```python
from build123d import *

# Parameters (mm, degrees)
SKETCH1_W                    = 14
SKETCH1_H                    = 8
SKETCH1_R                    = 2.5
BASE_FLANGE1_DEPTH           = 2
EDGE_FLANGE1_STRIP_W         = 9.4732
EDGE_FLANGE1_STRIP_H         = 2
EDGE_FLANGE1_STRIP_CUT_DEPTH = 8
EDGE_FLANGE1_DEPTH           = 8
EDGE_FLANGE1_PROFILE_W       = 8
EDGE_FLANGE1_PROFILE_H       = 11.2634
EDGE_FLANGE1_PROFILE_R       = 2.5
EDGE_FLANGE1_FLAT_DEPTH      = 2


# Sheet-metal steps are written as plain solids
with BuildPart() as part:
    # Sketch1 → Base-Flange1 (new body)
    with BuildSketch(Plane(origin=(0, 0, 0), x_dir=(1, 0, 0), z_dir=(0, 1, 0))):
        Rectangle(SKETCH1_W, SKETCH1_H)
        with Locations(Location((-2.5, 0, 0), (0, 0, 270))):
            Circle(SKETCH1_R, mode=Mode.SUBTRACT)
    extrude(amount=-BASE_FLANGE1_DEPTH)

    # Edge-Flange1 strip (across the edge) → Edge-Flange1 strip cut (cut)
    with BuildSketch(Plane(origin=(7, 0, 4), x_dir=(-1, 0, 0), z_dir=(0, 0, -1))):
        with Locations((-2, -1)):
            Rectangle(EDGE_FLANGE1_STRIP_W, EDGE_FLANGE1_STRIP_H)
    extrude(amount=EDGE_FLANGE1_STRIP_CUT_DEPTH, mode=Mode.SUBTRACT)

    # Edge-Flange1 bend section (across the edge) → Edge-Flange1 (add)
    with BuildSketch(Plane(origin=(7, 0, 4), x_dir=(-1, 0, 0), z_dir=(0, 0, -1))):
        with BuildLine():
            Line((0, 0.7366), (2, 0.7366))
            ThreePointArc((2, 0.7366), (2.215745145, 0.215745145), (2.7366, 0))
            Line((2.7366, 0), (2.7366, -2))
            ThreePointArc((2.7366, -2), (0.801531583, -1.198468417), (0, 0.7366))
        make_face()
    extrude(amount=EDGE_FLANGE1_DEPTH)

    # Edge-Flange1 profile (on flange) → Edge-Flange1 flat (add)
    with BuildSketch(Plane(origin=(7, 0, 0), x_dir=(0, 0, -1), z_dir=(1, 0, 0))):
        with Locations((0, 6.3683)):
            Rectangle(EDGE_FLANGE1_PROFILE_W, EDGE_FLANGE1_PROFILE_H)
        with Locations((0, 7.5)):
            Circle(EDGE_FLANGE1_PROFILE_R, mode=Mode.SUBTRACT)
    extrude(amount=-EDGE_FLANGE1_FLAT_DEPTH)


solid = part.part
```
Check sheet for the modelled part. Datum: model origin and axes. Units: mm. A direction names the side the tool comes from. Coordinates: 2 decimals unless noted, no trailing zeros. Order: outer loops, then holes, each group sorted by start corner. A loop starts at its lowest first (then second) coordinate and runs counter-clockwise, first axis right, second up. Notation, with made-up numbers: M 14.5,84.25 L 31.5,84.25 A3 ccw 31.5,89.25 Z; hole C 37.25,-21.75 d5. An arc over 180 degrees is marked long. Write each question's results on one line, items separated by ' | '. Start each with the question number.
1. Go/stop test with a flat-tipped pin: P1, Ø3, axis at y = 2, z = 1.5, coming from the -X side. Record where the tip stops, or that it passes through.
2. Cross-section at A-A on z = 0. Record the cut outline in (x, y).
3. Cross-section at B-B on y = 7.5. Record the cut outline in (x, z), and give its area (3 significant figures).
4. Mould release check, pull along X, two halves, no side actions. Record for faces 1 (the face through (6.01, 5.06, 0.54)), 2 (the face through (7, 5, 2)), 3 (the face through (-4.72, -0.99, 1.15)), 4 (the face through (-7, -1, 0)): +X half, -X half, draft (parallel to the pull), parting line (faces both ways), or undercut.
5. Cross-section at D-D on z = -2.75. Record the cut outline in (x, y), and give its area (3 significant figures).
6. Material ranges on probe 1 along Y at (x, z) = (2.25, 2.25); probe 2 along X at (y, z) = (4, 0.25); probe 3 along Y at (x, z) = (6, 0), recorded low to high.
7. Cross-section at C-C on x = -2.5. Record the cut outline in (y, z).
8. Access from +Z, -Z, +X, -X, +Y, -Y to the whole of each face (thin tool, end or side, straight path). Record for faces 5 (the face through (0, 0, -2)), 6 (the face through (2.6, -0.2, -4)).
Checks:
1) P1: stops at x = 4.96
2) outline: M -7,-2 L -5,-2 L -5,0 L -7,0 Z; M 0,-2 L 4.26,-2 A2.74 ccw 7,0.74 L 7,5 L 5,5 L 5,0.74 A0.74 cw 4.26,0 L 0,0 Z; M 5,10 L 7,10 L 7,12 L 5,12 Z
3) outline: M 5,-4 L 7,-4 L 7,-2.5 L 5,-2.5 Z; M 5,2.5 L 7,2.5 L 7,4 L 5,4 Z | area: 6.00 mm²
4) face 1: draft | face 2: +X half | face 3: undercut | face 4: -X half
5) outline: M -7,-2 L 4.26,-2 A2.74 ccw 7,0.74 L 7,12 L 5,12 L 5,0.74 A0.74 cw 4.26,0 L -7,0 Z | area: 50.5 mm²
6) probe 1: y = -2 to 0 | probe 2: x = 5 to 7 | probe 3: y = -1.38 to 5, 10 to 12
7) outline: M -2,-4 L 0,-4 L 0,-2.5 L -2,-2.5 Z; M -2,2.5 L 0,2.5 L 0,4 L -2,4 Z
8) face 5: +Z, -Z, -X, +Y | face 6: -Z, +X, -X, +Y, -Y
